from build123d import *

# Parameters (mm, degrees)
SALIENTE_EXTRUIR1_DEPTH = 6


with BuildPart() as part:
    # Croquis1 → Saliente-Extruir1 (new body)
    with BuildSketch(Plane(origin=(0, 0, 0), x_dir=(1, 0, 0), z_dir=(0, 1, 0))):
        with BuildLine():
            Line((-114.926621199, -5.742358079), (-122.476621199, -5.742358079))
            Line((-122.476621199, -5.742358079), (-122.476621199, -15.742358079))
            ThreePointArc((-122.476621199, -15.742358079), (-121.012155104, -19.277891985), (-117.476621199, -20.742358079))
            Line((-117.476621199, -20.742358079), (157.523378801, -20.742358079))
            ThreePointArc((157.523378801, -20.742358079), (161.058912707, -19.277891985), (162.523378801, -15.742358079))
            Line((162.523378801, -15.742358079), (162.523378801, -0.742358079))
            Line((162.523378801, -0.742358079), (162.523378801, 0.257641921))
            Line((162.523378801, 0.257641921), (154.223378801, 0.257641921))
            Line((154.223378801, 0.257641921), (153.723378801, 0.257641921))
            Line((153.723378801, 0.257641921), (153.723378801, 6.257641921))
            Line((153.723378801, 6.257641921), (131.723378801, 6.257641921))
            Line((131.723378801, 6.257641921), (131.723378801, 0.257641921))
            Line((131.723378801, 0.257641921), (131.223378801, 0.257641921))
            Line((131.223378801, 0.257641921), (101.873378801, 0.257641921))
            Line((101.873378801, 0.257641921), (101.873378801, -6.242583321))
            ThreePointArc((101.873378801, -6.242583321), (102.797983436, -6.770672857), (103.163716432, -7.770678689))
            Line((103.163716432, -7.770678689), (103.163716432, -9.320678689))
            ThreePointArc((103.163716432, -9.320678689), (102.975019602, -10.061862661), (102.454872975, -10.622583321))
            Line((102.454872975, -10.622583321), (102.285628043, -10.622583321))
            ThreePointArc((102.285628043, -10.622583321), (100.323378801, -11.435593306), (98.36112956, -10.622583321))
            Line((98.36112956, -10.622583321), (98.191884628, -10.622583321))
            ThreePointArc((98.191884628, -10.622583321), (97.671738001, -10.061862661), (97.483041171, -9.320678689))
            Line((97.483041171, -9.320678689), (97.483041171, -7.770678689))
            ThreePointArc((97.483041171, -7.770678689), (97.848774167, -6.770672857), (98.773378801, -6.242583321))
            Line((98.773378801, -6.242583321), (98.773378801, 0.257641921))
            Line((98.773378801, 0.257641921), (69.223378801, 0.257641921))
            Line((69.223378801, 0.257641921), (68.723378801, 0.257641921))
            Line((68.723378801, 0.257641921), (68.723378801, 6.257641921))
            Line((68.723378801, 6.257641921), (46.723378801, 6.257641921))
            Line((46.723378801, 6.257641921), (46.723378801, 0.257641921))
            Line((46.723378801, 0.257641921), (46.223378801, 0.257641921))
            Line((46.223378801, 0.257641921), (16.873378801, 0.257641921))
            Line((16.873378801, 0.257641921), (16.873378801, -6.242583321))
            ThreePointArc((16.873378801, -6.242583321), (17.797983436, -6.770672857), (18.163716432, -7.770678689))
            Line((18.163716432, -7.770678689), (18.163716432, -9.320678689))
            ThreePointArc((18.163716432, -9.320678689), (17.975019602, -10.061862661), (17.454872975, -10.622583321))
            Line((17.454872975, -10.622583321), (17.285628043, -10.622583321))
            ThreePointArc((17.285628043, -10.622583321), (15.323378801, -11.435593306), (13.36112956, -10.622583321))
            Line((13.36112956, -10.622583321), (13.191884628, -10.622583321))
            ThreePointArc((13.191884628, -10.622583321), (12.671738001, -10.061862661), (12.483041171, -9.320678689))
            Line((12.483041171, -9.320678689), (12.483041171, -7.770678689))
            ThreePointArc((12.483041171, -7.770678689), (12.848774167, -6.770672857), (13.773378801, -6.242583321))
            Line((13.773378801, -6.242583321), (13.773378801, 0.257641921))
            Line((13.773378801, 0.257641921), (-14.776621199, 0.257641921))
            Line((-14.776621199, 0.257641921), (-15.776621199, 0.257641921))
            Line((-15.776621199, 0.257641921), (-16.276621199, 0.257641921))
            Line((-16.276621199, 0.257641921), (-16.276621199, 6.257641921))
            Line((-16.276621199, 6.257641921), (-38.276621199, 6.257641921))
            Line((-38.276621199, 6.257641921), (-38.276621199, 0.257641921))
            Line((-38.276621199, 0.257641921), (-38.776621199, 0.257641921))
            Line((-38.776621199, 0.257641921), (-39.776621199, 0.257641921))
            Line((-39.776621199, 0.257641921), (-68.126621199, 0.257641921))
            Line((-68.126621199, 0.257641921), (-68.126621199, -6.242583321))
            ThreePointArc((-68.126621199, -6.242583321), (-67.202016564, -6.770672857), (-66.836283568, -7.770678689))
            Line((-66.836283568, -7.770678689), (-66.836283568, -9.320678689))
            ThreePointArc((-66.836283568, -9.320678689), (-67.024980398, -10.061862661), (-67.545127025, -10.622583321))
            Line((-67.545127025, -10.622583321), (-67.714371957, -10.622583321))
            ThreePointArc((-67.714371957, -10.622583321), (-69.676621199, -11.435593306), (-71.63887044, -10.622583321))
            Line((-71.63887044, -10.622583321), (-71.808115372, -10.622583321))
            ThreePointArc((-71.808115372, -10.622583321), (-72.328261999, -10.061862661), (-72.516958829, -9.320678689))
            Line((-72.516958829, -9.320678689), (-72.516958829, -7.770678689))
            ThreePointArc((-72.516958829, -7.770678689), (-72.151225833, -6.770672857), (-71.226621199, -6.242583321))
            Line((-71.226621199, -6.242583321), (-71.226621199, 0.257641921))
            Line((-71.226621199, 0.257641921), (-83.776621199, 0.257641921))
            Line((-83.776621199, 0.257641921), (-83.776621199, -5.742358079))
            Line((-83.776621199, -5.742358079), (-90.476621199, -5.742358079))
            Line((-90.476621199, -5.742358079), (-91.476621199, -5.742358079))
            Line((-91.476621199, -5.742358079), (-91.976621199, -5.742358079))
            Line((-91.976621199, -5.742358079), (-91.976621199, 6.257641921))
            Line((-91.976621199, 6.257641921), (-103.976621199, 6.257641921))
            Line((-103.976621199, 6.257641921), (-103.976621199, -5.742358079))
            Line((-103.976621199, -5.742358079), (-104.476621199, -5.742358079))
            Line((-104.476621199, -5.742358079), (-105.476621199, -5.742358079))
            Line((-105.476621199, -5.742358079), (-111.826621199, -5.742358079))
            Line((-111.826621199, -5.742358079), (-111.826621199, -12.242583321))
            ThreePointArc((-111.826621199, -12.242583321), (-110.902016564, -12.770672857), (-110.536283568, -13.770678689))
            Line((-110.536283568, -13.770678689), (-110.536283568, -15.320678689))
            ThreePointArc((-110.536283568, -15.320678689), (-110.724980398, -16.061862661), (-111.245127025, -16.622583321))
            Line((-111.245127025, -16.622583321), (-111.414371957, -16.622583321))
            ThreePointArc((-111.414371957, -16.622583321), (-113.376621199, -17.435593306), (-115.33887044, -16.622583321))
            Line((-115.33887044, -16.622583321), (-115.508115372, -16.622583321))
            ThreePointArc((-115.508115372, -16.622583321), (-116.028261999, -16.061862661), (-116.216958829, -15.320678689))
            Line((-116.216958829, -15.320678689), (-116.216958829, -13.770678689))
            ThreePointArc((-116.216958829, -13.770678689), (-115.851225833, -12.770672857), (-114.926621199, -12.242583321))
            Line((-114.926621199, -12.242583321), (-114.926621199, -5.742358079))
        make_face()
    extrude(amount=SALIENTE_EXTRUIR1_DEPTH)


solid = part.part
Model file for the job. Use its own axes, mm. A direction names the side the tool comes from. Give positions to 0.01 mm unless a question says otherwise; leave off trailing zeros. Loops run counter-clockwise (first coordinate to the right, second up) from the corner with the lowest first, then second, coordinate; pieces in that order, holes last. Notation, with made-up numbers: (-27, 61) -> (-19, 61) arc R30 cw to (-19, 89) -> close; hole circle Ø5 at (-27, 78.5). An arc over 180 degrees is marked (long way). Use a Markdown table: item, result. Add a question column.
(1) Slice it at A-A on x = -80. List the corners of the cut face in (y, z).
(2) Wall check: line 1 along X through (y, z) = (0.6, -4.75); line 2 along X through (y, z) = (4.9, 2.75); line 3 along X through (y, z) = (0.7, 13.5). Give the ranges that are in metal, low to high.
(3) Drop flat-ended pins along their axis: pin 1 Ø1.8 at (y, z) = (3.5, 0) entering from -X; pin 2 Ø1 at (x, z) = (-7, 9) entering from -Y. Give the stop position or say it passes through.
(4) Tool access for faces 1 (the flat face through (101.873, 3, 3)), 2 (the flat face through (-98, 3, -6.258)), 3 (the flat face through (158, 3, -0.258)): list every direction of +Z, -Z, +X, -X, +Y, -Y with a clear straight run to the whole face (end or side of a thin tool).
(5) Mould opens along X. For faces 4 (the flat face through (-38.277, 3, -3)), 5 (the cylindrical face through (161.02, 2.958, 19.317)), 6 (the flat face through (117, 3, -0.258)), 7 (the flat face through (18, 3, 20.742)) say: +X half, -X half, draft (parallel to the pull), parting line (faces both ways), or undercut.
Filled sheet:
| question | item | result |
|---|---|---|
| 1 | outline | (0, -0.26) -> (6, -0.26) -> (6, 20.74) -> (0, 20.74) -> close |
| 2 | line 1 | -103.98 to -91.98, -38.28 to -16.28, 46.72 to 68.72, 131.72 to 153.72 |
| 2 | line 2 | -103.98 to -91.98, -83.78 to -71.23, -68.13 to 13.77, 16.87 to 98.77, 101.87 to 162.52 |
| 2 | line 3 | -122.48 to -116.19, -110.56 to 162.52 |
| 3 | pin 1 | x = -103.98 |
| 3 | pin 2 | y = 0 |
| 4 | face 1 | -Z, +Y, -Y |
| 4 | face 2 | -Z, +X, -X, +Y, -Y |
| 4 | face 3 | -Z, +X, +Y, -Y |
| 5 | face 4 | undercut |
| 5 | face 5 | +X half |
| 5 | face 6 | undercut |
| 5 | face 7 | draft |
